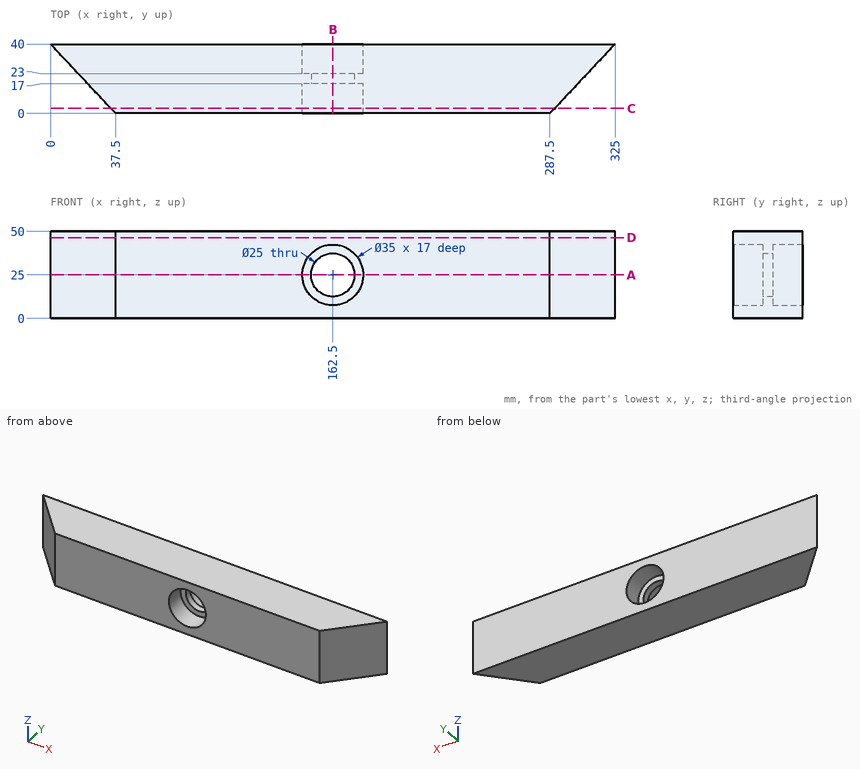
The drawing under review shows one solid part. Ordinate dimensions are in mm from its lowest x, y, z. Round coordinates to 2 decimals unless told otherwise and drop trailing zeros. Loops run counter-clockwise (first coordinate to the right, second up) from the corner with the lowest first, then second, coordinate; pieces in that order, holes last. Notation, with made-up numbers: (52.5, -21.75) - (101.5, -21.75) arc R34 cw to (101.5, 8.25) - close; hole circle Ø7 at (29.25, -15). An arc over 180 degrees is marked (long way). One line per question, with ' | ' between items.
1. We need section D-D, the plane z = 46.5. State the section outline as (x, y) points, and give its area (3 significant figures).
Results are:
outline: (0, 40) - (37.5, 0) - (287.5, 0) - (325, 40) - close | area: 11,500 mm²
2. For L1, parallel to Z at x = 162, y = 11; L2, parallel to Z at x = 162, y = 21; L3, parallel to Y at x = 163, z = 41.5, list the stretches that pass through material, from the lowest coordinate up. Write a range as [from, to].
Results are:
L1: z = [0, 7.51], [42.49, 50] | L2: z = [0, 12.51], [37.49, 50] | L3: y = [17, 23]
3. We need section B-B, the plane x = 162.5. State the section outline as (y, z) points, and give its area (3 significant figures).
Results are:
outline: (0, 0) - (40, 0) - (40, 7.5) - (23, 7.5) - (23, 12.5) - (17, 12.5) - (17, 7.5) - (0, 7.5) - close; (0, 42.5) - (17, 42.5) - (17, 37.5) - (23, 37.5) - (23, 42.5) - (40, 42.5) - (40, 50) - (0, 50) - close | area: 660 mm²
4. We need section C-C, the plane y = 3. State the section outline as (x, z) points, and give its area (3 significant figures).
Results are:
outline: (34.69, 0) - (290.31, 0) - (290.31, 50) - (34.69, 50) - close; hole circle Ø35 at (162.5, 25) | area: 11,800 mm²
5. Clearance check with flat-ended pins moving along their axes: P1, Ø10, axis at y = 33.5, z = 10.5, coming from the +X side; P2, Ø17.5, axis at x = 156, z = 32.5, coming from the -Y side; P3, Ø1, axis at y = 24, z = 27.5, coming from the -X side; P4, Ø1.5, axis at y = 19.5, z = 30, coming from the +X side. State where each tip first meets the part, or that it passes through.
Results are:
P1: stops at x = 323.59 | P2: stops at y = 0 | P3: stops at x = 14.53 | P4: stops at x = 306.48
6. We need section A-A, the plane z = 25. State the section outline as (x, y) points.
Results are:
outline: (0, 40) - (37.5, 0) - (145, 0) - (145, 17) - (150, 17) - (150, 23) - (145, 23) - (145, 40) - close; (175, 17) - (180, 17) - (180, 0) - (287.5, 0) - (325, 40) - (180, 40) - (180, 23) - (175, 23) - close
